Geometry check sheet. Reference: the model listing, model coordinates, mm. A direction names the side the tool comes from. Round coordinates to 2 decimals unless told otherwise and drop trailing zeros. Loops run counter-clockwise (first coordinate to the right, second up) from the corner with the lowest first, then second, coordinate; pieces in that order, holes last. Notation, with made-up numbers: (31.5, -4.75) - (85.5, -4.75) arc R19 ccw to (85.5, 11.25) - close; hole circle Ø9 at (26, 59). An arc over 180 degrees is marked (long way). Answer in a Markdown table with one row per item. Add a question column.
```python
from build123d import *

# Parameters (mm, degrees)
SKETCH1_W                  = 58.42
SKETCH1_H                  = 38.1
BOSS_EXTRUDE1_DEPTH        = 50.8
BOSS_EXTRUDE3_DEPTH        = 17.78
SKETCH3_R                  = 10.0965
BOSS_EXTRUDE4_DEPTH        = 7.62
SKETCH8_R                  = 18
CUT_EXTRUDE2_DEPTH         = 91.06261211
M8X1_25_TAPPED_HOLE1_D     = 6.8
M8X1_25_TAPPED_HOLE1_DEPTH = 25.4
M8X1_25_TAPPED_HOLE1_TIP   = 2.042926105
CIRPATTERN2_COUNT          = 8


with BuildPart() as part:
    # Sketch1 → Boss-Extrude1 (new body)
    with BuildSketch(Plane(origin=(0, 0, 0), x_dir=(1, 0, 0), z_dir=(0, 1, 0))):
        Rectangle(SKETCH1_W, SKETCH1_H)
    extrude(amount=BOSS_EXTRUDE1_DEPTH)

    # Sketch2 → Boss-Extrude3 (add)
    with BuildSketch(Plane(origin=(0, 50.8, 0), x_dir=(-1, 0, 0), z_dir=(0, 1, 0))):
        with BuildLine():
            Line((29.21, -29.21), (29.21, -10.795))
            ThreePointArc((29.21, -10.795), (20.654589078, 9.859589078), (0, 18.415))
            ThreePointArc((0, 18.415), (-20.654589078, 9.859589078), (-29.21, -10.795))
            Line((-29.21, -10.795), (-29.21, -29.21))
            Line((-29.21, -29.21), (29.21, -29.21))
        make_face()
    extrude(amount=BOSS_EXTRUDE3_DEPTH)

    # Sketch3 → Boss-Extrude4 (add)
    with BuildSketch(Plane(origin=(0, 68.58, 0), x_dir=(-1, 0, 0), z_dir=(0, 1, 0))):
        with Locations(Location((0, -10.795, 0), (0, 0, 270))):
            Circle(SKETCH3_R)
    extrude(amount=BOSS_EXTRUDE4_DEPTH)

    # Sketch8 → Cut-Extrude2 (cut, through all)
    with BuildSketch(Plane(origin=(0, 0, -19.05), x_dir=(-1, 0, 0), z_dir=(0, 0, -1))):
        with Locations((0, 21.59)):
            Circle(SKETCH8_R)
    extrude(amount=-CUT_EXTRUDE2_DEPTH, mode=Mode.SUBTRACT)

    # M8x1.25 Tapped Hole1
    with Locations(Plane(origin=(0, 76.2, 0), x_dir=(-1, 0, 0), z_dir=(0, 1, 0))):
        with Locations((0, -10.795)):
            Hole(M8X1_25_TAPPED_HOLE1_D / 2, depth=M8X1_25_TAPPED_HOLE1_DEPTH)
            with Locations((0, 0, -(M8X1_25_TAPPED_HOLE1_DEPTH + M8X1_25_TAPPED_HOLE1_TIP / 2))):  # 118° drill point
                Cone(0, M8X1_25_TAPPED_HOLE1_D / 2, M8X1_25_TAPPED_HOLE1_TIP, mode=Mode.SUBTRACT)

    # Sketch13 → 1/4-20 Tapped Hole1 (revolve, cut)
    with BuildSketch(Plane(origin=(-23.5, 21.59, -19.05), x_dir=(0, 1, 0), z_dir=(1, 0, 0))):
        Polygon((0, 0), (0, 20.583816902), (2.5527, 19.05), (2.5527, 0.635), (3.1877, 0), align=None)
    f_1_4_20_tapped_hole1 = revolve(axis=Axis((-23.5, 21.59, -25.4), (0, 0, 1)), mode=Mode.SUBTRACT)

    # CirPattern2: 1/4-20 Tapped Hole1 ×8 about axis, 2 skipped
    cirpattern2_axis = Axis((0, 21.59, 0), (0, 0, -1))
    add([f_1_4_20_tapped_hole1.rotate(cirpattern2_axis, i * 360 / CIRPATTERN2_COUNT) for i in range(1, CIRPATTERN2_COUNT) if i not in (2, 6)], mode=Mode.SUBTRACT)

    # Mirror2: 1/4-20 Tapped Hole1 across plane
    add(f_1_4_20_tapped_hole1.mirror(Plane.XY), mode=Mode.SUBTRACT)

    # Mirror2 copy 1 sketch → Mirror2 copy 1 (revolve, cut)
    with BuildSketch(Plane(origin=(-16.617009358, 38.207009358, 19.05), x_dir=(0.7071067811865475, 0.7071067811865476, 0), z_dir=(0.7071067811865476, -0.7071067811865475, 0))):
        Polygon((0, 0), (0, -20.583816902), (2.5527, -19.05), (2.5527, -0.635), (3.1877, 0), align=None)
    revolve(axis=Axis((-16.617009358, 38.207009358, 25.4), (0, 0, 1)), mode=Mode.SUBTRACT)

    # Mirror2 copy 2 sketch → Mirror2 copy 2 (revolve, cut)
    with BuildSketch(Plane(origin=(16.617009358, 38.207009358, 19.05), x_dir=(0.7071067811865476, -0.7071067811865475, 0), z_dir=(-0.7071067811865475, -0.7071067811865476, 0))):
        Polygon((0, 0), (0, -20.583816902), (2.5527, -19.05), (2.5527, -0.635), (3.1877, 0), align=None)
    revolve(axis=Axis((16.617009358, 38.207009358, 25.4), (0, 0, 1)), mode=Mode.SUBTRACT)

    # Mirror2 copy 3 sketch → Mirror2 copy 3 (revolve, cut)
    with BuildSketch(Plane(origin=(23.5, 21.59, 19.05), x_dir=(0, -1, 0), z_dir=(-1, 0, 0))):
        Polygon((0, 0), (0, -20.583816902), (2.5527, -19.05), (2.5527, -0.635), (3.1877, 0), align=None)
    revolve(axis=Axis((23.5, 21.59, 25.4), (0, 0, 1)), mode=Mode.SUBTRACT)

    # Mirror2 copy 4 sketch → Mirror2 copy 4 (revolve, cut)
    with BuildSketch(Plane(origin=(16.617009358, 4.972990642, 19.05), x_dir=(-0.7071067811865475, -0.7071067811865477, 0), z_dir=(-0.7071067811865477, 0.7071067811865475, 0))):
        Polygon((0, 0), (0, -20.583816902), (2.5527, -19.05), (2.5527, -0.635), (3.1877, 0), align=None)
    revolve(axis=Axis((16.617009358, 4.972990642, 25.4), (0, 0, 1)), mode=Mode.SUBTRACT)

    # Mirror2 copy 5 sketch → Mirror2 copy 5 (revolve, cut)
    with BuildSketch(Plane(origin=(-16.617009358, 4.972990642, 19.05), x_dir=(-0.7071067811865477, 0.7071067811865474, 0), z_dir=(0.7071067811865474, 0.7071067811865477, 0))):
        Polygon((0, 0), (0, -20.583816902), (2.5527, -19.05), (2.5527, -0.635), (3.1877, 0), align=None)
    revolve(axis=Axis((-16.617009358, 4.972990642, 25.4), (0, 0, 1)), mode=Mode.SUBTRACT)


solid = part.part
```
Q1. Cross-section at B-B, the plane x = -23.5. Enter the section's corners in (y, z) (3 decimals).
Q2. Cross-section at A-A, the plane y = 61. Enter the section's corners in (x, z) (3 decimals), plus the area to 3 significant figures.
Q3. Depth check by flat-ended pin: P1, Ø10, axis at x = -5.5, y = 64.5, coming from the +Z side; P2, Ø8, axis at x = -13.5, z = -22.5, coming from the -Y side; P3, Ø15, axis at x = -4.5, z = 8, coming from the +Y side; P4, Ø1, axis at x = 7.5, y = 48, coming from the -Z side. Enter the tip coordinate at first touch or a pass-through.
Q4. Scan lines: line 1 (Y direction, x = -23.5, z = -5); line 2 (Y direction, x = 0, z = -2); line 3 (X direction, y = 23.5, z = 10). Record each from-to range of solid material in increasing order. Write a range as from..to.
Q5. Release check for a two-part mould opening along Z. For faces 1 (the cylindrical face through (-0.443, 63.322, -7.424)), 2 (the flat face through (0, 42, 19.05)), 3 (the cylindrical face through (-6.82, 72.34, -3.35)), 4 (the flat face through (-29.21, 26, 0)) record: +Z half, -Z half, draft (parallel to the pull), parting line (faces both ways), or undercut.
Q6. Cross-section at D-D, the plane y = 42.5. Enter the section's corners in (x, z).
Q7. Cross-section at C-C, the plane z = 16.5. Enter the section's corners in (x, y).
Q8. Set-up check for faces 5 (the flat face through (-4.5, 50.8, 18.4)), 6 (the flat face through (0, 60, -29.21)), 7 (the flat face through (0, 50.8, -24)): record each of +Z, -Z, +X, -X, +Y, -Y from which the full face is reachable in a straight line by a thin tool's end or side.
Check sheet entries:
| question | item | result |
|---|---|---|
| 1 | outline | (0, -19.05) - (18.402, -19.05) - (19.037, -18.415) - (19.037, 18.415) - (18.402, 19.05) - (0, 19.05) - close; (24.143, -18.415) - (24.778, -19.05) - (50.8, -19.05) - (50.8, -29.21) - (68.58, -29.21) - (68.58, 6.554) - (50.8, 6.554) - (50.8, 19.05) - (24.778, 19.05) - (24.143, 18.415) - close |
| 2 | outline | (-29.21, -29.21) - (29.21, -29.21) - (29.21, -10.795) arc R29.21 ccw to (-29.21, -10.795) - close; hole circle Ø6.8 at (0, -10.795) |
| 2 | area | 2,380 mm² |
| 3 | P1 | z = 18.41 |
| 3 | P2 | y = 0 |
| 3 | P3 | y = 68.58 |
| 3 | P4 | z = -19.05 |
| 4 | line 1 | 0..19.04, 24.14..68.58 |
| 4 | line 2 | 0..3.59, 39.59..76.2 |
| 4 | line 3 | -29.21..-25.19, -21.81..-17.9, 17.9..21.81, 25.19..29.21 |
| 5 | face 1 | undercut |
| 5 | face 2 | +Z half |
| 5 | face 3 | parting line |
| 5 | face 4 | draft |
| 6 | outline | (-29.21, -19.05) - (29.21, -19.05) - (29.21, 19.05) - (-29.21, 19.05) - close |
| 7 | outline | (-29.21, 0) - (29.21, 0) - (29.21, 50.8) - (10.4, 50.8) - (10.4, 68.58) - (-10.4, 68.58) - (-10.4, 50.8) - (-29.21, 50.8) - close; hole circle Ø5.11 at (-23.5, 21.59); hole circle Ø5.11 at (-16.62, 4.97); hole circle Ø5.11 at (-16.62, 38.21); hole circle Ø36 at (0, 21.59); hole circle Ø5.11 at (16.62, 4.97); hole circle Ø5.11 at (16.62, 38.21); hole circle Ø5.11 at (23.5, 21.59) |
| 8 | face 5 | +Z, +Y |
| 8 | face 6 | -Z, +X, -X, +Y, -Y |
| 8 | face 7 | -Z, +X, -X, -Y |
